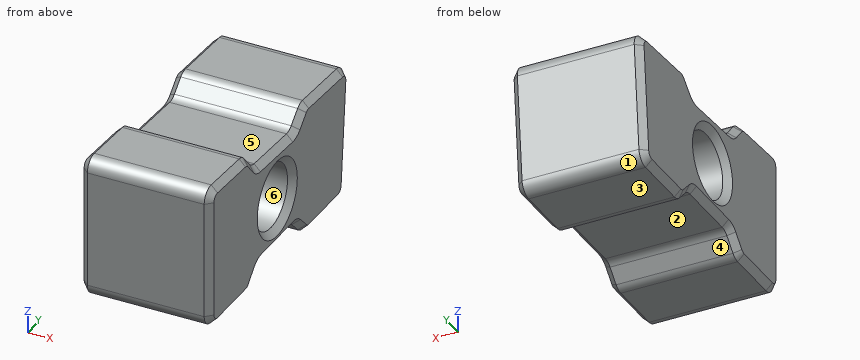
from build123d import *

# Parameters (mm, degrees)
SKETCH_R     = 2.505
PAD_DEPTH    = 10
FILLET_R     = 1
CHAMFER_SIZE = 0.5


with BuildPart() as part:
    # Sketch → Pad (new body)
    with BuildSketch(Plane.YZ):
        Polygon((0, 0), (0, 11.094006), (5.666667, 10.797029), (7.086107, 9.220581), (12.756885, 8.923388), (14.333333, 10.342828), (20.874887, 10), (20, 0), (14.333333, 0), (12.833333, 1.5), (7.166667, 1.5), (5.666667, 0), align=None)
        with Locations((10, 5.171414)):
            Circle(SKETCH_R, mode=Mode.SUBTRACT)
    extrude(amount=PAD_DEPTH)

    # Fillet
    fillet_edges = [part.edges().sort_by_distance(p)[0] for p in [
        (5, 0, 11.094006),
        (5, 5.666667, 10.797029),
        (5, 7.086107, 9.220581),
        (5, 12.756885, 8.923388),
        (5, 14.333333, 10.342828),
        (5, 20.874887, 10),
        (5, 0, 0),
        (5, 5.666667, 0),
        (5, 7.166667, 1.5),
        (5, 12.833333, 1.5),
        (5, 14.333333, 0),
        (5, 20, 0),
    ]]
    fillet(fillet_edges, radius=FILLET_R)

    # Chamfer
    chamfer_edges = [part.edges().sort_by_distance(p)[0] for p in [
        (0, 3.126227, 0),
        (0, 0.292893, 0.292893),
        (0, 5.635137, 0.07612),
        (0, 0, 5.520113),
        (0, 6.416667, 0.75),
        (0, 0.311645, 10.765601),
        (0, 7.198197, 1.42388),
        (0, 3.152678, 10.928782),
        (0, 10, 1.5),
        (0, 5.631196, 10.722663),
        (0, 12.801803, 1.42388),
        (0, 6.376387, 10.008805),
        (0, 13.583333, 0.75),
        (0, 7.121578, 9.294947),
        (0, 14.364863, 0.07612),
        (0, 9.921496, 9.071984),
        (0, 16.915608, 0),
        (0, 12.729382, 9.001054),
        (0, 19.759259, 0.262723),
        (0, 13.545109, 9.633108),
        (0, 20.432249, 4.940627),
        (0, 14.360836, 10.265162),
        (0, 20.543149, 9.711625),
        (0, 17.293877, 10.187673),
        (0, 7.495, 5.171414),
        (10, 3.126227, 0),
        (10, 0.292893, 0.292893),
        (10, 5.635137, 0.07612),
        (10, 0, 5.520113),
        (10, 6.416667, 0.75),
        (10, 0.311645, 10.765601),
        (10, 7.198197, 1.42388),
        (10, 3.152678, 10.928782),
        (10, 10, 1.5),
        (10, 5.631196, 10.722663),
        (10, 12.801803, 1.42388),
        (10, 6.376387, 10.008805),
        (10, 13.583333, 0.75),
        (10, 7.121578, 9.294947),
        (10, 14.364863, 0.07612),
        (10, 9.921496, 9.071984),
        (10, 16.915608, 0),
        (10, 12.729382, 9.001054),
        (10, 19.759259, 0.262723),
        (10, 13.545109, 9.633108),
        (10, 20.432249, 4.940627),
        (10, 14.360836, 10.265162),
        (10, 20.543149, 9.711625),
        (10, 17.293877, 10.187673),
        (10, 7.495, 5.171414),
    ]]
    chamfer(chamfer_edges, length=CHAMFER_SIZE)


solid = part.part
Model file for the job. Use its own axes, mm. Face numbers are marked on the shaded views. A direction names the side the tool comes from. Give positions to 0.01 mm unless a question says otherwise; leave off trailing zeros. Order: outer loops, then holes, each group sorted by start corner. A loop starts at its lowest first (then second) coordinate and runs counter-clockwise, first axis right, second up. Notation, with made-up numbers: M 76.25,-34 L 128.25,-34 A29 cw 128.25,-1 Z; hole C -27.5,18 d9. An arc over 180 degrees is marked long. Put each result on its own line as item: value. Start each with the question number.
(1) Tool access for the marked faces 4, 5 and 6: list every direction of +Z, -Z, +X, -X, +Y, -Y with a clear straight run to the whole face (end or side of a thin tool).
(2) Pin check, flat tips, straight feed: pin 1 Ø4 at (x, y) = (4.5, 9) entering from -Z; pin 2 Ø4 at (x, y) = (6.5, 12) entering from -Z; pin 3 Ø4 at (x, y) = (1, 15) entering from +Z. Stop position of each tip, or through.
(3) Drill centre lines: L1, parallel to Z at x = 7.5, y = 10; L2, parallel to Z at x = 5.25, y = 11.5; L3, parallel to Y at x = 7, z = 5.75. Where is each one in solid material? Low to high. Write a range as [from, to].
(4) Band-saw the part on B-B on x = 4.5. Give the cut face in (y, z) (3 decimals), then the cut area to 3 significant figures.
(5) Band-saw the part on A-A on y = 10. Give the cut face in (x, z).
(6) Band-saw the part on C-C on y = 3.5. Give the cut face in (x, z), then the cut area to 3 significant figures.
(7) Pull direction Y, two halves, no side cores. Call the marked faces 1, 2 and 3: released by +Y, released by -Y, zero draft, split by the parting line, or undercut.
Results below:
1. face 4: -Z, +X, -X
1. face 5: +Z, +X, -X
1. face 6: +X, -X
2. pin 1: stops at z = 1.31
2. pin 2: stops at z = 0.33
2. pin 3: stops at z = 10.32
3. L1: z = [1.5, 2.67], [7.68, 9.07]
3. L2: z = [1.5, 3.17], [7.18, 8.99]
3. L3: y = [0, 7.56], [12.44, 20.5]
4. outline: M 0,1 A1 ccw 1,0 L 5.252,0 A1 ccw 5.96,0.293 L 6.874,1.207 A1 cw 7.581,1.5 L 12.419,1.5 A1 cw 13.126,1.207 L 14.04,0.293 A1 ccw 14.748,0 L 19.084,0 A1 ccw 20.08,0.913 L 20.785,8.968 A1 ccw 19.841,10.054 L 14.747,10.321 A1 ccw 14.026,10.066 L 13.065,9.201 A1 cw 12.343,8.945 L 7.5,9.199 A1 cw 6.809,9.528 L 5.944,10.489 A1 ccw 5.253,10.819 L 1.052,11.039 A1 ccw 0,10.04 Z; hole C 10,5.171 d5.01
4. area: 174 mm2
5. outline: M 0,2 L 0.5,1.5 L 9.5,1.5 L 10,2 L 10,2.17 L 9.5,2.67 L 0.5,2.67 L 0,2.17 Z; M 0,8.18 L 0.5,7.68 L 9.5,7.68 L 10,8.18 L 10,8.57 L 9.5,9.07 L 0.5,9.07 L 0,8.57 Z
6. outline: M 0,0.5 L 0.5,0 L 9.5,0 L 10,0.5 L 10,10.41 L 9.5,10.91 L 0.5,10.91 L 0,10.41 Z
6. area: 109 mm2
7. face 1: released by +Y
7. face 2: undercut
7. face 3: zero draft
